from build123d import *

# Parameters (mm, degrees)
SKETCH1_W           = 646
SKETCH1_H           = 646
BOSS_EXTRUDE1_DEPTH = 5
SKETCH2_R           = 4
CUT_EXTRUDE1_DEPTH  = 6
CHAMFER1_SIZE       = 3


with BuildPart() as part:
    # Sketch1 → Boss-Extrude1 (new body)
    with BuildSketch(Plane(origin=(0, 0, 0), x_dir=(1, 0, 0), z_dir=(0, 1, 0))):
        Rectangle(SKETCH1_W, SKETCH1_H)
    extrude(amount=BOSS_EXTRUDE1_DEPTH)

    # Sketch2 → Cut-Extrude1 (cut, through all)
    with BuildSketch(Plane(origin=(0, 5, 0), x_dir=(1, 0, 0), z_dir=(0, 1, 0))):
        with Locations((-223, -298)):
            Circle(SKETCH2_R)
        with Locations((223, -298)):
            Circle(SKETCH2_R)
        with Locations((-298, -223)):
            Circle(SKETCH2_R)
        with Locations((298, -223)):
            Circle(SKETCH2_R)
        with Locations((298, 223)):
            Circle(SKETCH2_R)
        with Locations((223, 298)):
            Circle(SKETCH2_R)
        with Locations((-223, 298)):
            Circle(SKETCH2_R)
        with Locations((-298, 223)):
            Circle(SKETCH2_R)
    extrude(amount=-CUT_EXTRUDE1_DEPTH, mode=Mode.SUBTRACT)

    # Chamfer1
    chamfer1_edges = [part.edges().sort_by_distance(p)[0] for p in [
        (-227, 5, 298),
        (219, 5, 298),
        (-302, 5, 223),
        (294, 5, 223),
        (294, 5, -223),
        (219, 5, -298),
        (-227, 5, -298),
        (-302, 5, -223),
    ]]
    chamfer(chamfer1_edges, length=CHAMFER1_SIZE)


solid = part.part
Verification items for the finished model (mm, model axes). Give positions to 0.01 mm unless a question says otherwise; leave off trailing zeros. Write item = value, one per line. Start each with the question number.
Q1. Mould release check, pull along Z, two halves, no side actions. Record for faces 1 (the face through (-302.142, 2.146, 222.818)), 2 (the face through (-5, 5, -5)): released by +Z, released by -Z, zero draft, split by the parting line, or undercut.
Q2. Depth check by flat-ended pin: P1, Ø9, axis at x = 223, z = 298, coming from the +Y side; P2, Ø5, axis at x = -298, z = -223, coming from the -Y side. Enter the tip coordinate at first touch or a pass-through.
Q3. Thickness scan on line 1 (Z direction, x = -298, y = 1.3); line 2 (X direction, y = 1.45, z = -223). Record the ranges inside material, lowest first.
Answer key:
q1.face_1 = undercut
q1.face_2 = zero draft
q2.P1 = 2.5
q2.P2 = through
q3.line_1 = -323 to -227, -219 to 219, 227 to 323
q3.line_2 = -323 to -302, -294 to 294, 302 to 323
